Autodesk Inventor part; units mm, degrees
ref_plane "YZ Plane" through (0, 0, 0) normal (1, 0, 0) x (0, 1, 0)
ref_plane "XZ Plane" through (0, 0, 0) normal (0, 1, 0) x (-1, 0, 0)
ref_plane "XY Plane" through (0, 0, 0) normal (0, 0, 1) x (1, 0, 0)
sketch "Sketch1" plane through (0, 0, 0) normal (0, 1, 0) x (-1, 0, 0)
  line L0 (-1.7321, -3) -> (-3.4641, 0)
  line L1 (-3.4641, 0) -> (-1.7321, 3)
  line L2 (-1.7321, 3) -> (1.7321, 3)
  line L3 (1.7321, 3) -> (3.4641, 0)
  line L4 (3.4641, 0) -> (1.7321, -3)
  line L5 (1.7321, -3) -> (-1.7321, -3)
  point P0 (0, 0)
  point P1 (0, 0)
  point P2 (0, 0)
  dimension "d0" = 3
extrude "Extrusion1" add sketch "Sketch1" along normal blind 15
hole "Hole2" at (0, 0, 0) direction (0, 1, 0) diameter 3.242 depth 11.8 tip angle 118
sketch "Sketch3" plane through (0, 15, 0) normal (0, 1, 0) x (1, 0, 0)
  circle A0 centre (0, 0) radius 2
  dimension "d17" = 4
extrude "Extrusion2" add sketch "Sketch3" along normal blind 6
thread "Thread1"
chamfer "Chamfer1" distance 0.7 angle 45 1 edges at (-2, 21, 0)
properties part number "StandoffM4x15B" material "Brass, Soft Yellow"
Source: CAD feature listing. Evaluate the final solid. Frame: model axes, mm. A direction names the side the tool comes from. Coordinates: 2 decimals unless noted, no trailing zeros. Order: outer loops, then holes, each group sorted by start corner. A loop starts at its lowest first (then second) coordinate and runs counter-clockwise, first axis right, second up. Notation, with made-up numbers: M 88,84.25 L 137,84.25 A12 ccw 137,97.25 Z; hole C 29,82 d2. An arc over 180 degrees is marked long. Write each question's results on one line, items separated by ' | '. Start each with the question number.
1. Section C-C, the plane x = 2.5. Return the cut outline in (y, z).
2. Section A-A, the plane y = 18.5. Return the cut outline in (x, z).
3. Section B-B, the plane y = 12. Return the cut outline in (x, z).
4. Section D-D, the plane z = 2.3. Return the cut outline in (x, y), then the cut area to 3 significant figures.
5. Draft query along Z for faces 4 (the face through (-2.6, 7.4, -1.5)), 5 (the face through (0, 18, -2)), 6 (the face through (-0.275, 12.605, 0.061)). Return one class per face: +Z half, -Z half, draft (parallel to the pull), parting line (faces both ways), or undercut.
6. Pin query (flat end, axial travel): pin 1 (1.5 mm diameter, centred on y = 11.5, z = 0.5, fed in from -X). Return the tip coordinate at first contact, or that it passes through.
7. Material intervals for L1, parallel to Z at x = 0, y = 9; L2, parallel to Y at x = 2.75, z = 0.9; L3, parallel to X at y = 4.25, z = 0.4, sorted ascending.
8. Reachability of faces 1 (the face through (-1, 15, 2)), 2 (the face through (1.438, 5.983, -0.748)), 3 (the face through (-1.5, 0, 1.4)) from +Z, -Z, +X, -X, +Y, -Y: full face, straight path, thin tool, end or side. Return the list, or none.
Solution:
1) outline: M 0,-1.67 L 15,-1.67 L 15,1.67 L 0,1.67 Z
2) outline: C 0,0 d4
3) outline: M -3.46,0 L -1.73,-3 L 1.73,-3 L 3.46,0 L 1.73,3 L -1.73,3 Z; hole C 0,0 d2.58
4) outline: M -2.14,0 L 2.14,0 L 2.14,15 L -2.14,15 Z | area: 64.1 mm²
5) face 4: -Z half | face 5: parting line | face 6: undercut
6) pin 1: x = -3.46
7) L1: -3 to -1.62, 1.62 to 3 | L2: 0 to 15 | L3: -3.23 to -1.57, 1.57 to 3.23
8) face 1: +Y | face 2: -Y | face 3: +Z, -Z, +X, -X, -Y
